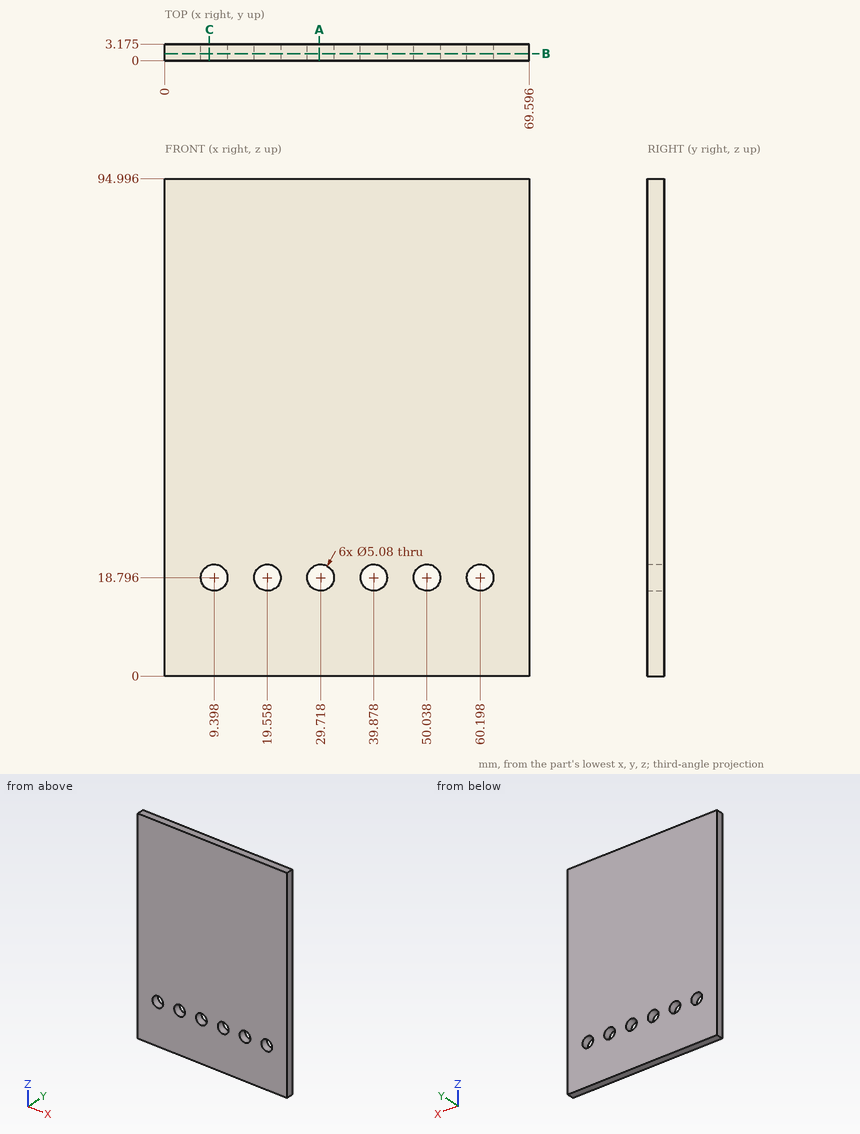
Here's the drawing with two shaded views (mm, measured from the low corner). I have some questions. Coordinates: 2 decimals unless noted, no trailing zeros. Write each loop counter-clockwise with the first axis right and the second up, starting at its lowest first coordinate (ties: lowest second). Pieces come first, ordered by that corner, then holes.
Item 1: Will this pin go through, and if not, where does the flat tip stop? pin 1 (3 mm diameter, centred on x = 29.718, z = 18.796, fed in from -Y).
Item 2: I want a section at B-B on y = 1.35. Write out the boundary of the cut face in (x, z).
Item 3: If I drill on line 1 (Z direction, x = 42, y = 2.25); line 2 (Z direction, x = 28.5, y = 1.7), over which ranges is the centre line in solid material (lowest first)?
Item 4: I want a section at A-A on x = 29.5. Write out the boundary of the cut face in (y, z) (3 decimals), and give its area (3 significant figures).
Item 5: I want a section at C-C on x = 8.5. Write out the boundary of the cut face in (y, z) (3 decimals).
Findings below:
1. pin 1: passes through
2. outline: (0, 0) - (69.6, 0) - (69.6, 95) - (0, 95) - close; hole circle Ø5.08 at (9.4, 18.8); hole circle Ø5.08 at (19.56, 18.8); hole circle Ø5.08 at (29.72, 18.8); hole circle Ø5.08 at (39.88, 18.8); hole circle Ø5.08 at (50.04, 18.8); hole circle Ø5.08 at (60.2, 18.8)
3. line 1: z = 0 to 17.4, 20.19 to 95
3. line 2: z = 0 to 16.57, 21.02 to 95
4. outline: (0, 0) - (3.175, 0) - (3.175, 16.265) - (0, 16.265) - close; (0, 21.327) - (3.175, 21.327) - (3.175, 94.996) - (0, 94.996) - close
4. area: 286 mm2
5. outline: (0, 0) - (3.175, 0) - (3.175, 16.42) - (0, 16.42) - close; (0, 21.172) - (3.175, 21.172) - (3.175, 94.996) - (0, 94.996) - close
